Check sheet for the modelled part. Datum: model origin and axes. Units: mm. Face numbers are marked on the shaded views. Round coordinates to 2 decimals unless told otherwise and drop trailing zeros. Order: outer loops, then holes, each group sorted by start corner. A loop starts at its lowest first (then second) coordinate and runs counter-clockwise, first axis right, second up. Notation, with made-up numbers: (54, -6.75) -> (105, -6.75) arc R31 ccw to (105, 21.25) -> close; hole circle Ø6 at (5, 21). An arc over 180 degrees is marked (long way). Answer in a Markdown table with one row per item.
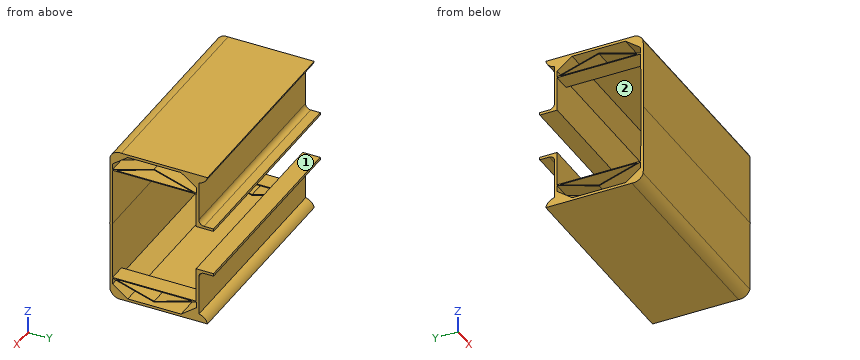
```python
from build123d import *

# Parameters (mm, degrees)
F1_DEPTH = 60
F3_DEPTH = 10


# Not quite as in the source:
# - a feature names something its author has since deleted; it is built from what else it names


with BuildPart() as f1:
    # F0 (on Right) → F1 (new body)
    with BuildSketch(Plane.YZ):
        with BuildLine():
            Line((24.139301102, -43.2624049591), (15.4307844338, -49.7964277864))
            Line((15.4307844338, -49.7964277864), (-15.1525954085, -49.7964277864))
            Line((-15.1525954085, -49.7964277864), (-23.8611120767, -43.2624049591))
            Line((-23.8611120767, -43.2624049591), (-24.0144912707, -6.2964277864))
            Line((-24.0144912707, -6.2964277864), (-25.5145041825, -6.2964277864))
            Line((-25.5145041825, -6.2964277864), (-25.3453201973, -47.0715236276))
            ThreePointArc((-25.3453201973, -47.0715236276), (-22.8573335388, -50.3682627369), (-18.8327744315, -51.2964277864))
            Line((-18.8327744315, -51.2964277864), (30.5735625925, -51.2964277864))
            ThreePointArc((30.5735625925, -51.2964277864), (28.8360021374, -48.2011592055), (25.6532847593, -46.6294995689))
            Line((25.6532847593, -46.6294995689), (25.5585974487, -23.8088752761))
            ThreePointArc((25.5585974487, -23.8088752761), (26.432854985, -21.6795128694), (28.5585716253, -20.7964277864))
            Line((28.5585716253, -20.7964277864), (34.0398614944, -20.7964277864))
            Line((34.0398614944, -20.7964277864), (34.0398614944, -19.2964277864))
            Line((34.0398614944, -19.2964277864), (24.0398614944, -19.2964277864))
            Line((24.0398614944, -19.2964277864), (24.139301102, -43.2624049591))
        make_face()
    extrude(amount=F1_DEPTH)

    # F2 (on face) → F3 (join)
    with BuildSketch(Plane.YZ.offset(60)):
        Polygon((24.1226036063, -39.2381352516), (-23.8778095724, -39.2381352516), (-23.8757047067, -39.7454297089), (-0.0007817785, -47.1604929972), (24.1247084719, -39.7454297089), align=None)
        Polygon((0, -46.6294995689), (-22.1652372944, -39.7454297089), (22.3978614654, -39.7454297089), align=None, mode=Mode.SUBTRACT)
    extrude(amount=-F3_DEPTH)

    # F4: F1 across plane


with BuildPart() as f1_1:
    add(f1.part)
    add(f1.part.mirror(Plane.YZ))

    # F5: F1 across face


with BuildPart() as f1_2:
    add(f1_1.part)
    add(f1_1.part.mirror(Plane(origin=(0, -24.7644977266, -6.2964277864), x_dir=(1, 0, 0), z_dir=(0, 0, 1))))


solid = f1_2.part
```
(1) Section check A-A on x = 24. Record the boundary of the cut face in (y, z).
Solutions:
| item | result |
|---|---|
| outline | (-25.51, -6.3) -> (-25.35, -47.07) arc R6.04 ccw to (-18.83, -51.3) -> (30.57, -51.3) arc R6 ccw to (25.65, -46.63) -> (25.56, -23.81) arc R3 cw to (28.56, -20.8) -> (34.04, -20.8) -> (34.04, -19.3) -> (24.04, -19.3) -> (24.14, -43.26) -> (15.43, -49.8) -> (-15.15, -49.8) -> (-23.86, -43.26) -> (-24.01, -6.3) -> (-23.86, 30.67) -> (-15.15, 37.2) -> (15.43, 37.2) -> (24.14, 30.67) -> (24.04, 6.7) -> (34.04, 6.7) -> (34.04, 8.2) -> (28.56, 8.2) arc R3 cw to (25.56, 11.22) -> (25.65, 34.04) arc R6 ccw to (30.57, 38.7) -> (-18.83, 38.7) arc R6.04 ccw to (-25.35, 34.48) -> close |
(2) Section check D-D on z = 4. Record the boundary of the cut face in (x, y), plus the area to 3 significant figures.
Solutions:
| item | result |
|---|---|
| outline | (-60, -25.47) -> (60, -25.47) -> (60, -23.97) -> (-60, -23.97) -> close |
| area | 180 mm^2 |
(3) Draft check along Y on the marked faces 1 and 2. Enter one of: pulls with the +Y half, pulls with the -Y half, needs draft (parallel to the pull), parting line crosses it, or undercut.
Solutions:
| item | result |
|---|---|
| face 1 | needs draft |
| face 2 | undercut |
(4) Section check B-B on z = -35. Record the boundary of the cut face in (x, y).
Solutions:
| item | result |
|---|---|
| outline | (-60, -25.4) -> (60, -25.4) -> (60, -23.9) -> (-60, -23.9) -> close; (-60, 24.11) -> (60, 24.11) -> (60, 25.61) -> (-60, 25.61) -> close |
(5) Section check C-C on y = -17. Give the number of separate pieces and of enclosed holes in the cut face, plus the area to 3 significant figures.
Solutions:
| item | result |
|---|---|
| separate pieces | 10 |
| enclosed holes | 0 |
| area | 734 mm^2 |
(6) Scan lines: probe 1 along Y at (x, z) = (28, 30); probe 2 along Z at (x, y) = (-9, 4.5); probe 3 along Z at (x, y) = (-50, 25). Record each from-to range of solid material in increasing order. Write a range as from..to.
Solutions:
| item | result |
|---|---|
| probe 1 | -25.36..-23.86, 24.14..25.64 |
| probe 2 | -51.3..-49.8, 37.2..38.7 |
| probe 3 | -51.3..-19.3, 6.7..38.7 |
(7) Depth check by flat-ended pin: pin 1 Ø5 at (x, y) = (13, 30.5) entering from -Z; pin 2 Ø15 at (x, y) = (-7, 5.5) entering from +Z; pin 3 Ø2.5 at (y, z) = (4.5, 32) entering from -X; pin 4 Ø5 at (x, z) = (-43.5, 2.5) entering from -Y. Enter the tip coordinate at first touch or a pass-through.
Solutions:
| item | result |
|---|---|
| pin 1 | z = -51.3 |
| pin 2 | z = 38.7 |
| pin 3 | x = -60 |
| pin 4 | y = -25.49 |
